```python
from build123d import *

# Parameters (mm, degrees)
F0_R     = 5.5
F0_R_2   = 4.6625
F1_DEPTH = 2.5
F2_R     = 4.8625
F3_DEPTH = 1.5


with BuildPart() as f1:
    # F0 (on Top) → F1 (new body, symmetric)
    with BuildSketch(Plane.XY):
        with BuildLine():
            Line((24.408629, 2), (16.881943, 2))
            ThreePointArc((16.881943, 2), (15.799858, 6.274111), (13.655032, 10.126209))
            Line((13.655032, 10.126209), (20.975247, 22.805193))
            ThreePointArc((20.975247, 22.805193), (11.7375, 20.329946), (9.262253, 29.567693))
            Line((9.262253, 29.567693), (1.942038, 16.888709))
            ThreePointArc((1.942038, 16.888709), (-2.466389, 16.820134), (-6.708921, 15.620192))
            Line((-6.708921, 15.620192), (-10.472264, 22.138493))
            Line((-10.472264, 22.138493), (-12.204315, 21.138493))
            Line((-12.204315, 21.138493), (-13.936365, 20.138493))
            Line((-13.936365, 20.138493), (-10.173022, 13.620192))
            ThreePointArc((-10.173022, 13.620192), (-13.333469, 10.546023), (-15.59707, 6.7625))
            Line((-15.59707, 6.7625), (-30.2375, 6.7625))
            ThreePointArc((-30.2375, 6.7625), (-25.45569, 4.78181), (-23.475, 0))
            ThreePointArc((-23.475, 0), (-25.45569, -4.78181), (-30.2375, -6.7625))
            Line((-30.2375, -6.7625), (-15.59707, -6.7625))
            ThreePointArc((-15.59707, -6.7625), (-13.333469, -10.546023), (-10.173022, -13.620192))
            Line((-10.173022, -13.620192), (-13.936365, -20.138493))
            Line((-13.936365, -20.138493), (-12.204315, -21.138493))
            Line((-12.204315, -21.138493), (-10.472264, -22.138493))
            Line((-10.472264, -22.138493), (-6.708921, -15.620192))
            ThreePointArc((-6.708921, -15.620192), (-2.466389, -16.820134), (1.942038, -16.888709))
            Line((1.942038, -16.888709), (9.262253, -29.567693))
            ThreePointArc((9.262253, -29.567693), (11.7375, -20.329946), (20.975247, -22.805193))
            Line((20.975247, -22.805193), (13.655032, -10.126209))
            ThreePointArc((13.655032, -10.126209), (15.799858, -6.274111), (16.881943, -2))
            Line((16.881943, -2), (24.408629, -2))
            Line((24.408629, -2), (24.408629, 0))
            Line((24.408629, 0), (24.408629, 2))
        make_face()
        Circle(F0_R, mode=Mode.SUBTRACT)
        with BuildLine():
            ThreePointArc((9.262253, 29.567693), (11.7375, 20.329946), (20.975247, 22.805193))
            ThreePointArc((20.975247, 22.805193), (21.650823, 24.436179), (21.88125, 26.186443))
            ThreePointArc((21.88125, 26.186443), (16.869014, 32.718517), (9.262253, 29.567693))
        make_face()
        with Locations((15.11875, 26.186443)):
            Circle(F0_R_2, mode=Mode.SUBTRACT)
        with BuildLine():
            ThreePointArc((21.88125, -26.186443), (21.650823, -24.436179), (20.975247, -22.805193))
            ThreePointArc((20.975247, -22.805193), (11.7375, -20.329946), (9.262253, -29.567693))
            ThreePointArc((9.262253, -29.567693), (16.869014, -32.718517), (21.88125, -26.186443))
        make_face()
        with Locations((15.11875, -26.186443)):
            Circle(F0_R_2, mode=Mode.SUBTRACT)
        with BuildLine():
            ThreePointArc((-23.475, 0), (-25.45569, 4.78181), (-30.2375, 6.7625))
            ThreePointArc((-30.2375, 6.7625), (-37, 0), (-30.2375, -6.7625))
            ThreePointArc((-30.2375, -6.7625), (-25.45569, -4.78181), (-23.475, 0))
        make_face()
        with Locations((-30.2375, 0)):
            Circle(F0_R_2, mode=Mode.SUBTRACT)
    extrude(amount=F1_DEPTH, both=True)

    # F2 (on Top) → F3 (cut, symmetric)
    with BuildSketch(Plane.XY):
        with Locations((-30.2375, 0)):
            Circle(F2_R)
        with Locations((15.11875, 26.186443)):
            Circle(F2_R)
        with Locations((15.11875, -26.186443)):
            Circle(F2_R)
    extrude(amount=F3_DEPTH, both=True, mode=Mode.SUBTRACT)


solid = f1.part
```
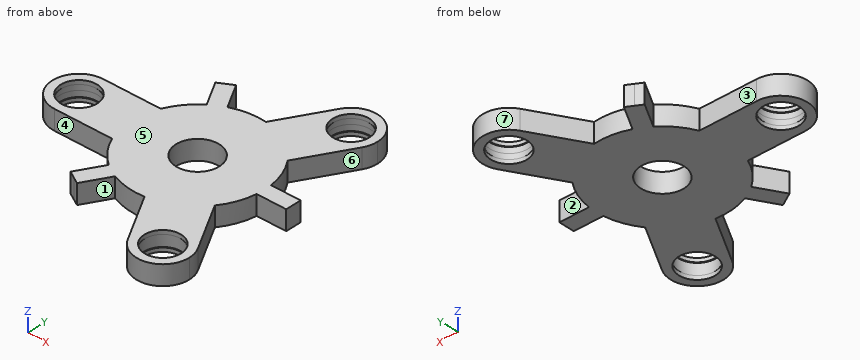
Geometry check sheet. Reference: the model listing, model coordinates, mm. Face numbers are marked on the shaded views. A direction names the side the tool comes from. Round coordinates to 2 decimals unless told otherwise and drop trailing zeros. Loops run counter-clockwise (first coordinate to the right, second up) from the corner with the lowest first, then second, coordinate; pieces in that order, holes last. Notation, with made-up numbers: M -27,84.5 L -10,84.5 A30 cw -10,119.5 Z; hole C -28,-1.75 d10. An arc over 180 degrees is marked long. Return JSON: item names as keys, results as strings. Group by question number.
(1) Section check B-B, the plane y = 0. Enter the section's corners in (x, z) (3 decimals), and give its area (3 significant figures).
(2) Section check D-D, the plane y = 8.5. Enter the section's corners in (x, z), and give its area (3 significant figures).
(3) Mould release check, pull along Y, two halves, no side actions. Record for the marked faces 5, 6 and 7: pulls with the +Y half, pulls with the -Y half, needs draft (parallel to the pull), parting line crosses it, or undercut.
(4) Section check C-C, the plane x = -13. Enter the section's corners in (y, z).
(5) Set-up check for the marked faces 1, 2, 3 and 4: record each of +Z, -Z, +X, -X, +Y, -Y from which the full face is reachable in a straight line by a thin tool's end or side.
(6) Scan lines: line 1 along Y through (x, z) = (15, 1.9); line 2 along X through (y, z) = (22, -0.45); line 3 along X through (y, z) = (-2.5, 1.05). Record each from-to range of solid material in increasing order. Write a range as [from, to].
(7) Go/stop test with flat-tipped pins: pin 1 (5.5 mm diameter, centred on x = 15.12, y = 26.19, fed in from +Z); pin 2 (15 mm diameter, centred on x = -30.24, y = 0, fed in from -Z); pin 3 (2 mm diameter, centred on x = 5.5, z = 1, fed in from -Y); pin 4 (1.5 mm diameter, centred on x = 19, z = -0.5, fed in from +Y). Record where each tip stops, or that it passes through.
(8) Section check A-A, the plane x = 0. Enter the section's corners in (y, z), and give its area (3 significant figures).
Data:
{
 "1": {"outline": "M -37,-2.5 L -34.9,-2.5 L -34.9,-1.5 L -35.1,-1.5 L -35.1,1.5 L -34.9,1.5 L -34.9,2.5 L -37,2.5 Z; M -25.575,-2.5 L -5.5,-2.5 L -5.5,2.5 L -25.575,2.5 L -25.575,1.5 L -25.375,1.5 L -25.375,-1.5 L -25.575,-1.5 Z; M 5.5,-2.5 L 24.409,-2.5 L 24.409,2.5 L 5.5,2.5 Z", "area": "204 mm²"},
 "2": {"outline": "M -14.72,-2.5 L 14.72,-2.5 L 14.72,2.5 L -14.72,2.5 Z", "area": "147 mm²"},
 "3": {"face 5": "needs draft", "face 6": "undercut", "face 7": "pulls with the +Y half"},
 "4": {"outline": "M -20.68,-2.5 L -18.52,-2.5 L -18.52,2.5 L -20.68,2.5 Z; M -10.95,-2.5 L 10.95,-2.5 L 10.95,2.5 L -10.95,2.5 Z; M 18.52,-2.5 L 20.68,-2.5 L 20.68,2.5 L 18.52,2.5 Z"},
 "5": {"face 1": "+Z, -Z, -Y", "face 2": "+Z, -Z, +X", "face 3": "+Z, -Z, -X, +Y", "face 4": "+Z, -Z, -X, -Y"},
 "6": {"line 1": "[-32.95, -30.85], [-21.53, -12.46], [-8, 8], [12.46, 21.53], [30.85, 32.95]", "line 2": "[-10.71, -10.39], [4.89, 12.65], [17.59, 20.51]", "line 3": "[-36.52, -34.41], [-26.07, -4.9], [4.9, 16.82]"},
 "7": {"pin 1": "through", "pin 2": "z = -2.5", "pin 3": "y = -24.78", "pin 4": "y = 32.18"},
 "8": {"outline": "M -17,-2.5 L -5.5,-2.5 L -5.5,2.5 L -17,2.5 Z; M 5.5,-2.5 L 17,-2.5 L 17,2.5 L 5.5,2.5 Z", "area": "115 mm²"}
}
